from build123d import *

# Parameters (mm, degrees)
F0_R     = 44
F1_DEPTH = 3
F3_W     = 25
F3_H     = 41
F6_R     = 25
F5_W     = 88
F5_H     = 88
F8_R     = 23.5
F9_DEPTH = 41


with BuildPart() as f1:
    # F0 (on Top) → F1 (new body)
    with BuildSketch(Plane.XY):
        Circle(F0_R)
    extrude(amount=F1_DEPTH)


with BuildPart() as f4:
    # F3 (on Front) → F4 (revolve)
    with BuildSketch(Plane.XZ):
        with Locations((12.5, 23.5)):
            Rectangle(F3_W, F3_H)
    revolve(axis=Axis((0, 0, 22), (0, 0, 1)))

    # F6 (on face) → F7 section 0
    with BuildSketch(Plane(origin=(0, 0, 3), x_dir=(1, 0, 0), z_dir=(0, 0, -1))):
        Circle(F6_R)
    # F5 (on Top) → F7 section 1
    with BuildSketch(Plane.XY):
        Rectangle(F5_W, F5_H)
    loft()

    # F8 (on face) → F9 (cut)
    with BuildSketch(Plane.XY.offset(44)):
        Circle(F8_R)
    extrude(amount=-F9_DEPTH, mode=Mode.SUBTRACT)


solid = f4.part
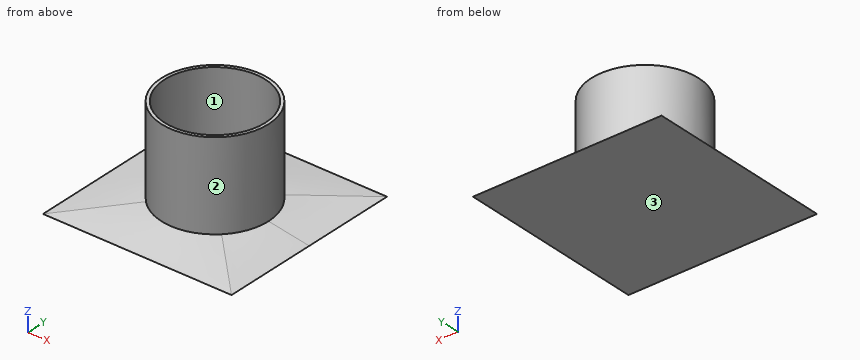
Could you check a few things on this model? Use its own coordinates, in mm. Face numbers are marked on the shaded views. Round coordinates to 2 decimals unless told otherwise and drop trailing zeros. Write each loop counter-clockwise with the first axis right and the second up, starting at its lowest first coordinate (ties: lowest second). Pieces come first, ordered by that corner, then holes. Notation, with made-up numbers: (-5.75, -8.5) - (51.25, -8.5) arc R8 cw to (51.25, -0.5) - close; hole circle Ø1 at (38.25, -15.5). An arc over 180 degrees is marked (long way). Use a Markdown table: item, result.
Q1. Please list where these lines run through material, in increasing order: L1, parallel to Y at x = 1, z = 10.5; L2, parallel to X at y = 0.5, z = 31.5 (3 decimals); L3, parallel to X at y = 20, z = 35.
Output values:
| item | result |
|---|---|
| L1 | -24.98 to -23.48, 23.48 to 24.98 |
| L2 | -24.995 to -23.495, 23.495 to 24.995 |
| L3 | -15 to -12.34, 12.34 to 15 |
Q2. I want a section at A-A (z = 11). List the corners of the cut face in (x, y) for me, plus the area to 3 significant figures.
Output values:
| item | result |
|---|---|
| outline | circle Ø50 at (0, 0); hole circle Ø47 at (0, 0) |
| area | 229 mm2 |
Q3. For pin 1 (1 mm diameter, centred on x = 13.5, z = 25, fed in from +Y); pin 2 (4 mm diameter, centred on x = 6.5, y = -6.5, fed in from +Z); pin 3 (1.5 mm diameter, centred on x = -16.5, z = 20.5, fed in from -Y), each with a flat end and sliding along its axis, tell me the tip position at first contact or that it passes through.
Output values:
| item | result |
|---|---|
| pin 1 | y = 21.35 |
| pin 2 | z = 3 |
| pin 3 | y = -19.41 |
Q4. Thinking about a two-plate mould opening in X: for the marked faces 1, 2 and 3, which applies, released by +X, released by -X, zero draft, split by the parting line, or undercut?
Output values:
| item | result |
|---|---|
| face 1 | undercut |
| face 2 | split by the parting line |
| face 3 | zero draft |
